Model file for the job. Use its own axes, mm. A direction names the side the tool comes from. Round coordinates to 2 decimals unless told otherwise and drop trailing zeros. Loops run counter-clockwise (first coordinate to the right, second up) from the corner with the lowest first, then second, coordinate; pieces in that order, holes last. Notation, with made-up numbers: M 87,80.25 L 104,80.25 A14 cw 104,87.25 Z; hole C 57,10 d2. An arc over 180 degrees is marked long. Answer in a Markdown table with one row per item.
from build123d import *

# Parameters (mm, degrees)
SKETCH1_R           = 49.53
BOSS_EXTRUDE1_DEPTH = 12.7
CUT_EXTRUDE1_DEPTH  = 72.188003203


with BuildPart() as part:
    # Sketch1 → Boss-Extrude1 (new body)
    with BuildSketch(Plane(origin=(0, 0, 0), x_dir=(1, 0, 0), z_dir=(0, 1, 0))):
        with Locations(Location((0, 0, 0), (0, 0, 270))):
            Circle(SKETCH1_R)
    extrude(amount=BOSS_EXTRUDE1_DEPTH)

    # Sketch2 → Cut-Extrude1 (cut, through all)
    with BuildSketch(Plane(origin=(0, 12.7, 0), x_dir=(1, 0, 0), z_dir=(0, 1, 0))):
        with BuildLine():
            Line((12.7, -34.169941281), (-12.7, -34.169941281))
            ThreePointArc((-12.7, -34.169941281), (-17.78, -29.089941281), (-12.7, -24.009941281))
            Line((-12.7, -24.009941281), (12.7, -24.009941281))
            ThreePointArc((12.7, -24.009941281), (17.78, -29.089941281), (12.7, -34.169941281))
        make_face()
        with BuildLine():
            Line((-12.7, 36.864035983), (12.7, 36.864035983))
            ThreePointArc((12.7, 36.864035983), (17.78, 31.784035983), (12.7, 26.704035983))
            Line((12.7, 26.704035983), (-12.7, 26.704035983))
            ThreePointArc((-12.7, 26.704035983), (-17.78, 31.784035983), (-12.7, 36.864035983))
        make_face()
    extrude(amount=-CUT_EXTRUDE1_DEPTH, mode=Mode.SUBTRACT)


solid = part.part
1. Tool access for faces 1 (the flat face through (1, 0, -1)), 2 (the cylindrical face through (-17.78, 6.44, 29.2)): list every direction of +Z, -Z, +X, -X, +Y, -Y with a clear straight run to the whole face (end or side of a thin tool).
Verdict:
| item | result |
|---|---|
| face 1 | +Z, -Z, +X, -X, -Y |
| face 2 | +Y, -Y |
2. Saw through at A-A (x = 0). Write the cut outline in (y, z), and give its area (4 significant figures).
Verdict:
| item | result |
|---|---|
| outline | M 0,-49.53 L 12.7,-49.53 L 12.7,-36.86 L 0,-36.86 Z; M 0,-26.7 L 12.7,-26.7 L 12.7,24.01 L 0,24.01 Z; M 0,34.17 L 12.7,34.17 L 12.7,49.53 L 0,49.53 Z |
| area | 1,000 mm² |
3. Saw through at D-D (x = 36). Write the cut outline in (y, z), and give its area (3 significant figures).
Verdict:
| item | result |
|---|---|
| outline | M 0,-34.02 L 12.7,-34.02 L 12.7,34.02 L 0,34.02 Z |
| area | 864 mm² |
4. Mould opens along Z. For faces 3 (the cylindrical face through (17.78, 6.44, -31.9)), 4 (the flat face through (0, 6, 34.17)), 5 (the cylindrical face through (14.88, 6.26, 47.24)), 6 (the flat face through (1, 12.7, -1)) say: +Z half, -Z half, draft (parallel to the pull), parting line (faces both ways), or undercut.
Verdict:
| item | result |
|---|---|
| face 3 | undercut |
| face 4 | undercut |
| face 5 | parting line |
| face 6 | draft |
5. Wall check: probe 1 along Z at (x, y) = (6.5, 8); probe 2 along Z at (x, y) = (-15.5, 10.5); probe 3 along X at (y, z) = (8, -34.5). Give the ranges that are in metal, low to high.
Verdict:
| item | result |
|---|---|
| probe 1 | z = -49.1 to -36.86, -26.7 to 24.01, 34.17 to 49.1 |
| probe 2 | z = -47.04 to -36.02, -27.55 to 24.85, 33.33 to 47.04 |
| probe 3 | x = -35.54 to -16.99, 16.99 to 35.54 |
6. Saw through at B-B (y = 5.5). Write the cut outline in (x, z).
Verdict:
| item | result |
|---|---|
| outline | C 0,0 d99.06; hole M -12.7,-36.86 L 12.7,-36.86 A5.08 ccw 12.7,-26.7 L -12.7,-26.7 A5.08 ccw Z; hole M -12.7,24.01 L 12.7,24.01 A5.08 ccw 12.7,34.17 L -12.7,34.17 A5.08 ccw Z |
7. Saw through at C-C (z = 33). Write the cut outline in (x, y).
Verdict:
| item | result |
|---|---|
| outline | M -36.94,0 L -15.94,0 L -15.94,12.7 L -36.94,12.7 Z; M 15.94,0 L 36.94,0 L 36.94,12.7 L 15.94,12.7 Z |
8. Pin check, flat tips, straight feed: pin 1 (1.5 mm diameter, centred on x = -35.5, y = 9, fed in from +Z); pin 2 (1 mm diameter, centred on x = 6, y = 4.5, fed in from +Z); pin 3 (1.5 mm diameter, centred on x = 22.5, y = 11.5, fed in from +Z). Stop position of each tip, or through.
Verdict:
| item | result |
|---|---|
| pin 1 | stops at z = 35.29 |
| pin 2 | stops at z = 49.22 |
| pin 3 | stops at z = 44.5 |
